For this review, take the finished solid that the model builds, in its own axes (mm). Face numbers are marked on the shaded views. Give positions to 0.01 mm unless a question says otherwise; leave off trailing zeros. Loops run counter-clockwise (first coordinate to the right, second up) from the corner with the lowest first, then second, coordinate; pieces in that order, holes last. Notation, with made-up numbers: (-13, 35.25) - (24, 35.25) arc R18 ccw to (24, 68.25) - close; hole circle Ø3 at (-25, -15.5). An arc over 180 degrees is marked (long way). Put each result on its own line as item: value. Start each with the question number.
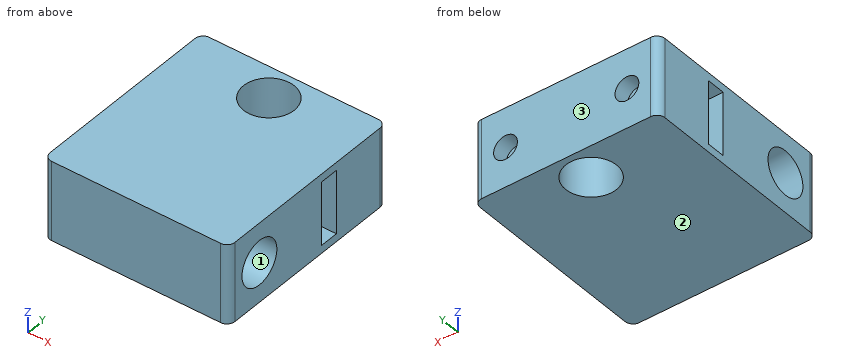
from build123d import *

# Parameters (mm, degrees)
SKETCH1_W           = 29.59652174
SKETCH1_H           = 50.8
SKETCH1_R           = 4.064
BOSS_EXTRUDE1_DEPTH = 12.7
SKETCH2_W           = 10.16
SKETCH2_H           = 3
CUT_EXTRUDE1_DEPTH  = 30.48
SKETCH3_R           = 3.556
CUT_EXTRUDE2_DEPTH  = 45.72
SKETCH4_R           = 1.143
CUT_EXTRUDE3_DEPTH  = 14.290068122
SKETCH5_R           = 1.905
CUT_EXTRUDE4_DEPTH  = 5.08
SKETCH7_W           = 12.7
SKETCH7_H           = 11.050531838
CUT_EXTRUDE5_DEPTH  = 62.484
SKETCH8_W           = 29.59652174
SKETCH8_H           = 2.54
CUT_EXTRUDE6_DEPTH  = 62.484
SKETCH9_W           = 12.7
SKETCH9_H           = 5.08
CUT_EXTRUDE7_DEPTH  = 62.484
FILLET1_R           = 1.27


with BuildPart() as part:
    # Sketch1 → Boss-Extrude1 (new body)
    with BuildSketch(Plane.XY):
        Rectangle(SKETCH1_W, SKETCH1_H)
        with Locations((0, 17.78)):
            Circle(SKETCH1_R, mode=Mode.SUBTRACT)
    extrude(amount=BOSS_EXTRUDE1_DEPTH)

    # Sketch2 → Cut-Extrude1 (cut)
    with BuildSketch(Plane.ZY.offset(14.79826087)):
        with Locations((6.35, 11.2)):
            Rectangle(SKETCH2_W, SKETCH2_H)
    extrude(amount=-CUT_EXTRUDE1_DEPTH, mode=Mode.SUBTRACT)

    # Sketch3 → Cut-Extrude2 (cut)
    with BuildSketch(Plane.ZY.offset(14.79826087)):
        with Locations((6.35, -3)):
            Circle(SKETCH3_R)
    extrude(amount=-CUT_EXTRUDE2_DEPTH, mode=Mode.SUBTRACT)

    # Sketch4 → Cut-Extrude3 (cut)
    with BuildSketch(Plane(origin=(0, 25.4, 0), x_dir=(1, 0, 0), z_dir=(0, 1, 0))):
        with Locations((9.71826087, -6.35)):
            Circle(SKETCH4_R)
        with Locations((-9.71826087, -6.35)):
            Circle(SKETCH4_R)
    extrude(amount=-CUT_EXTRUDE3_DEPTH, mode=Mode.SUBTRACT)

    # Sketch5 → Cut-Extrude4 (cut)
    with BuildSketch(Plane(origin=(0, 25.4, 0), x_dir=(1, 0, 0), z_dir=(0, 1, 0))):
        with Locations((-9.71826087, -6.35)):
            Circle(SKETCH5_R)
        with Locations((9.71826087, -6.35)):
            Circle(SKETCH5_R)
    extrude(amount=-CUT_EXTRUDE4_DEPTH, mode=Mode.SUBTRACT)

    # Sketch7 → Cut-Extrude5 (cut)
    with BuildSketch(Plane.ZY.offset(14.79826087)):
        with Locations((6.35, -19.874734081)):
            Rectangle(SKETCH7_W, SKETCH7_H)
    extrude(amount=-CUT_EXTRUDE5_DEPTH, mode=Mode.SUBTRACT)

    # Sketch8 → Cut-Extrude6 (cut)
    with BuildSketch(Plane.XY.offset(12.7)):
        with Locations((0, 24.13)):
            Rectangle(SKETCH8_W, SKETCH8_H)
    extrude(amount=-CUT_EXTRUDE6_DEPTH, mode=Mode.SUBTRACT)

    # Sketch9 → Cut-Extrude7 (cut)
    with BuildSketch(Plane.ZY.offset(14.79826087)):
        with Locations((6.35, -11.809468162)):
            Rectangle(SKETCH9_W, SKETCH9_H)
    extrude(amount=-CUT_EXTRUDE7_DEPTH, mode=Mode.SUBTRACT)

    # Fillet1
    fillet1_edges = [part.edges().sort_by_distance(p)[0] for p in [
        (14.79826087, -9.269468162, 6.35),
        (-14.79826087, -9.269468162, 6.35),
        (-14.79826087, 22.86, 6.35),
        (14.79826087, 22.86, 6.35),
    ]]
    fillet(fillet1_edges, radius=FILLET1_R)


solid = part.part
1) Take a section at C-C on y = 17.78. State the section outline as (x, z) points.
2) Insertion check: P1, Ø2.5, axis at x = 9.72, z = 6.35, coming from the +Y side; P2, Ø4.5, axis at y = -3, z = 6.35, coming from the +X side. Each pin has a flat end and moves straight along its axis. Give the tip position at first contact, or say it passes through.
3) Take a section at D-D on y = -3. State the section outline as (x, z) points.
4) Wall thickness on probe 1 along Y at (x, z) = (3, 2.75); probe 2 along X at (y, z) = (16.75, 6.35); probe 3 along Z at (x, y) = (1.5, 11): over which ranges is each line inside the solid? List them lowest first.
5) Take a section at A-A on z = 2. State the section outline as (x, y) points, and give its area (3 significant figures).
6) Take a section at B-B on x = 0. State the section outline as (y, z) points.
7) Mouldability with a two-part tool opening along Y and no side actions: class the marked faces 1, 2 and 3 as released by +Y, released by -Y, zero draft, split by the parting line, or undercut.
Answers follow:
1. outline: (-14.8, 0) - (-4.06, 0) - (-4.06, 12.7) - (-14.8, 12.7) - close; (4.06, 0) - (14.8, 0) - (14.8, 12.7) - (4.06, 12.7) - close; hole circle Ø2.29 at (-9.72, 6.35); hole circle Ø2.29 at (9.72, 6.35)
2. P1: y = 20.32
2. P2: through
3. outline: (-14.8, 0) - (14.8, 0) - (14.8, 2.79) - (-14.8, 2.79) - close; (-14.8, 9.91) - (14.8, 9.91) - (14.8, 12.7) - (-14.8, 12.7) - close
4. probe 1: -9.27 to 9.7, 12.7 to 15.04, 20.52 to 22.86
4. probe 2: -14.8 to -10.86, -8.58 to -3.93, 3.93 to 8.58, 10.86 to 14.8
4. probe 3: 0 to 1.27, 11.43 to 12.7
5. outline: (-14.8, -8) arc R1.27 ccw to (-13.53, -9.27) - (13.53, -9.27) arc R1.27 ccw to (14.8, -8) - (14.8, 9.7) - (-14.8, 9.7) - close; (-14.8, 12.7) - (14.8, 12.7) - (14.8, 21.59) arc R1.27 ccw to (13.53, 22.86) - (-13.53, 22.86) arc R1.27 ccw to (-14.8, 21.59) - close; hole circle Ø8.13 at (0, 17.78)
5. area: 809 mm2
6. outline: (-9.27, 0) - (13.72, 0) - (13.72, 12.7) - (-9.27, 12.7) - close; (21.84, 0) - (22.86, 0) - (22.86, 12.7) - (21.84, 12.7) - close; hole circle Ø7.11 at (-3, 6.35); hole (9.7, 1.27) - (12.7, 1.27) - (12.7, 11.43) - (9.7, 11.43) - close
7. face 1: undercut
7. face 2: zero draft
7. face 3: released by +Y
